```python
from build123d import *

# Parameters (mm, degrees)
SKETCH014_W     = 200
SKETCH014_H     = 200
PAD007_DEPTH    = 12.7
SKETCH015_W     = 329.815369
SKETCH015_H     = 292.155731
POCKET002_DEPTH = 13
FILLET_R        = 10


with BuildPart() as part:
    # Sketch014 → Pad007 (new body)
    with BuildSketch(Plane.XY):
        with Locations((100, -100)):
            Rectangle(SKETCH014_W, SKETCH014_H)
    extrude(amount=PAD007_DEPTH)

    # Sketch015 (on Face6 of Pad007) → Pocket002 (cut)
    with BuildSketch(Plane.XY.offset(12.7)):
        with Locations((191.907684, -173.077866)):
            Rectangle(SKETCH015_W, SKETCH015_H)
    extrude(amount=-POCKET002_DEPTH, mode=Mode.SUBTRACT)

    # Fillet
    fillet_edges = [part.edges().sort_by_distance(p)[0] for p in [
        (27, -27, 6.35),
    ]]
    fillet(fillet_edges, radius=FILLET_R)


with BuildPart() as part_1:
    # Body008 placement: moved
    add(part.part.moved(Location((0, -22, 231))))


solid = part_1.part
```
Here's how the part is built. I have some questions about the finished solid (model axes, mm). A direction names the side the tool comes from. Give positions to 0.01 mm unless a question says otherwise; leave off trailing zeros. Loops run counter-clockwise (first coordinate to the right, second up) from the corner with the lowest first, then second, coordinate; pieces in that order, holes last. Notation, with made-up numbers: M 17,14.25 L 73,14.25 A9 cw 73,20.25 Z; hole C 12.5,29 d6. An arc over 180 degrees is marked long. Use one line per item in the form item = value. Start each with the question number.
Q1. If we section it at C-C (y = -153.5): Write out the boundary of the cut face in (x, z).
Q2. I need wall thicknesses on line 1 along X through (y, z) = (-166.5, 232.25); line 2 along Y through (x, z) = (72.5, 240.75); line 3 along Y through (x, z) = (29, 236). Which ranges of each line are inside material? Lowest first, please.
Q3. If we section it at A-A (z = 233.5): Write out the boundary of the cut face in (x, y).
Q4. Will these pins go through, and if not, where does the flat tip stop? pin 1 Ø1 at (x, z) = (123.5, 234.5) entering from -Y; pin 2 Ø3 at (y, z) = (-153, 241.5) entering from +X.
Q5. If we section it at B-B (x = 31): Write out the boundary of the cut face in (y, z).
Q6. Which directions (+Z, -Z, +X, -X, +Y, -Y) give clear straight access to the entire face, cutting with the end or side of a thin tool? Please do faces 1 (the flat face through (200, -36, 237)), 2 (the flat face through (27, -142, 237)).
Taken from the geometry:
q1.outline = M 0,231 L 27,231 L 27,243.7 L 0,243.7 Z
q2.line_1 = 0 to 27
q2.line_2 = -49 to -22
q2.line_3 = -53 to -22
q3.outline = M 0,-222 L 27,-222 L 27,-59 A10 cw 37,-49 L 200,-49 L 200,-22 L 0,-22 Z
q4.pin_1 = -49
q4.pin_2 = 27
q5.outline = M -51,231 L -22,231 L -22,243.7 L -51,243.7 Z
q6.face_1 = +Z, -Z, +X, +Y, -Y
q6.face_2 = +Z, -Z, +X, -Y
